For this review, take the finished solid that the model builds, in its own axes (mm). Coordinates: 2 decimals unless noted, no trailing zeros. Order: outer loops, then holes, each group sorted by start corner. A loop starts at its lowest first (then second) coordinate and runs counter-clockwise, first axis right, second up. Notation, with made-up numbers: M -6.5,56.25 L 49.5,56.25 A15 cw 49.5,64.25 Z; hole C 51,70 d2. An arc over 180 degrees is marked long. Use CSV: the item, a comma, the result in double quotes.
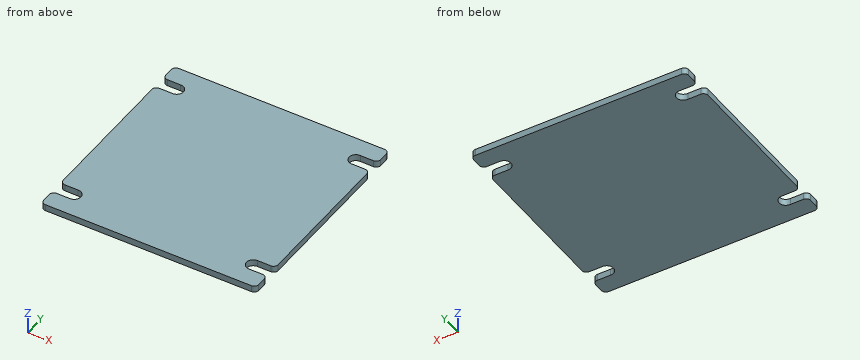
```python
from build123d import *

# Parameters (mm, degrees)
F1_DEPTH = 9.271
F2_R     = 6.35


with BuildPart() as f1:
    # F0 (on Top) → F1 (new body)
    with BuildSketch(Plane.XY):
        with BuildLine():
            Line((-152.4, -152.4), (0, -152.4))
            Line((0, -152.4), (152.4, -152.4))
            Line((152.4, -152.4), (152.4, -126.969507))
            Line((152.4, -126.969507), (127.761554, -126.969507))
            ThreePointArc((127.761554, -126.969507), (117.475854, -117.602548), (127.507025, -107.963504))
            Line((127.507025, -107.963504), (152.4, -107.963504))
            Line((152.4, -107.963504), (152.4, 107.980493))
            Line((152.4, 107.980493), (127.761554, 107.980493))
            ThreePointArc((127.761554, 107.980493), (117.475854, 117.347452), (127.507025, 126.986496))
            Line((127.507025, 126.986496), (152.4, 126.986496))
            Line((152.4, 126.986496), (152.4, 152.4))
            Line((152.4, 152.4), (0, 152.4))
            Line((0, 152.4), (-152.4, 152.4))
            Line((-152.4, 152.4), (-152.4, 126.986496))
            Line((-152.4, 126.986496), (-127.507025, 126.986496))
            ThreePointArc((-127.507025, 126.986496), (-117.475854, 117.347452), (-127.761554, 107.980493))
            Line((-127.761554, 107.980493), (-152.4, 107.980493))
            Line((-152.4, 107.980493), (-152.4, -107.963504))
            Line((-152.4, -107.963504), (-127.507025, -107.963504))
            ThreePointArc((-127.507025, -107.963504), (-117.475854, -117.602548), (-127.761554, -126.969507))
            Line((-127.761554, -126.969507), (-152.4, -126.969507))
            Line((-152.4, -126.969507), (-152.4, -152.4))
        make_face()
    extrude(amount=F1_DEPTH)

    # F2
    f2_edges = [f1.edges().sort_by_distance(p)[0] for p in [
        (-152.4, 152.4, 4.6355),
        (152.4, 152.4, 4.6355),
        (152.4, -152.4, 4.6355),
        (-152.4, -152.4, 4.6355),
        (152.4, -126.969507, 4.6355),
        (152.4, -107.963504, 4.6355),
        (152.4, 107.980493, 4.6355),
        (152.4, 126.986496, 4.6355),
        (-152.4, -107.963504, 4.6355),
        (-152.4, 126.986496, 4.6355),
        (-152.4, -126.969507, 4.6355),
        (-152.4, 107.980493, 4.6355),
    ]]
    fillet(f2_edges, radius=F2_R)


solid = f1.part
```
Item 1: To check wall thickness, follow line 1 along X through (y, z) = (117, 3.25); line 2 along Y through (x, z) = (122, 5.25); line 3 along Y through (x, z) = (-122.5, 9). State the ranges of each line that lie inside material, in increasing order. Write a range as [from, to].
Solutions:
line 1,"[-117.49, 117.49]"
line 2,"[-152.4, -125.58], [-109.37, 109.37], [125.58, 152.4]"
line 3,"[-152.4, -125.87], [-109.08, 109.08], [125.87, 152.4]"
Item 2: Add section A-A on x = -132.5. State the section outline as (y, z) points, and give its area (3 significant figures).
Solutions:
outline,"M -152.4,0 L -126.97,0 L -126.97,9.27 L -152.4,9.27 Z; M -107.96,0 L 107.98,0 L 107.98,9.27 L -107.96,9.27 Z; M 126.99,0 L 152.4,0 L 152.4,9.27 L 126.99,9.27 Z"
area,"2,470 mm^2"
Item 3: Add section C-C on y = 112. State the section outline as (x, z) points, and give its area (3 significant figures).
Solutions:
outline,"M -119.21,0 L 119.21,0 L 119.21,9.27 L -119.21,9.27 Z"
area,"2,210 mm^2"
Item 4: Clearance check with a flat-ended pin moving along its axis: pin 1 Ø5 at (y, z) = (121, 6.5) entering from +X. State where the tip first meets the part, or that it passes through.
Solutions:
pin 1,"x = 119.62"
